from build123d import *

# Parameters (mm, degrees)
F0_R     = 54.998868
F1_DEPTH = 30
F2_R     = 49.998868
F2_R_2   = 48.998866
F3_DEPTH = 3
F4_R     = 49.998868
F4_R_2   = 48.998866
F5_DEPTH = 3


with BuildPart() as f1:
    # F0 (on Top) → F1 (new body)
    with BuildSketch(Plane.XY):
        Circle(F0_R)
    extrude(amount=F1_DEPTH)

    # F2 (on face) → F3 (join)
    with BuildSketch(Plane(origin=(0, 0, 0), x_dir=(1, 0, 0), z_dir=(0, 0, -1))):
        Circle(F2_R)
        Circle(F2_R_2, mode=Mode.SUBTRACT)
    extrude(amount=F3_DEPTH)

    # F4 (on face) → F5 (join)
    with BuildSketch(Plane.XY.offset(30)):
        Circle(F4_R)
        Circle(F4_R_2, mode=Mode.SUBTRACT)
    extrude(amount=F5_DEPTH)


solid = f1.part
The model under review builds one solid part; all positions refer to its coordinate system, in mm. A direction names the side the tool comes from. Give positions to 0.01 mm unless a question says otherwise; leave off trailing zeros. Loops run counter-clockwise (first coordinate to the right, second up) from the corner with the lowest first, then second, coordinate; pieces in that order, holes last. Notation, with made-up numbers: (-8.5, 43.25) -> (33.5, 43.25) arc R24 ccw to (33.5, 67.25) -> close; hole circle Ø2 at (77, 33). An arc over 180 degrees is marked (long way). Put each result on its own line as item: value. Start each with the question number.
1. Clearance check with flat-ended pins moving along their axes: P1, Ø1, axis at x = 9, z = 7, coming from the -Y side; P2, Ø12, axis at y = -25, z = 6.5, coming from the +X side; P3, Ø1, axis at y = -39, z = 3.5, coming from the +X side. State where each tip first meets the part, or that it passes through.
2. We need section A-A on y = 0. State the section outline as (x, z) points, then the cut area to 3 significant figures.
3. Wall thickness on probe 1 along Y at (x, z) = (0, -1); probe 2 along Z at (x, y) = (14, 38.5): over which ranges is each line inside the solid? List them lowest first.
4. We need section C-C on z = 26.5. State the section outline as (x, y) points, then the cut area to 3 significant figures.
5. For faces 1 (the face through (-1, 1, 30)), 2 (the face through (33, 37, -3)), 3 (the face through (12, -49, 0)), list the 3-axis set-ups (+Z, -Z, +X, -X, +Y, -Y) from which the entire face can be reached by the end or side of a thin tool; tool diameter is ignored.
6. Mouldability with a two-part tool opening along X and no side actions: class faces 4 (the face through (12, -49, 30)), 5 (the face through (-6.509, -49.573, -1.479)), 6 (the face through (-10.622, 47.834, -1.479)) as released by +X, released by -X, zero draft, split by the parting line, or undercut.
Determined:
1. P1: y = -54.34
1. P2: x = 51.61
1. P3: x = 39.28
2. outline: (-55, 0) -> (-50, 0) -> (-50, -3) -> (-49, -3) -> (-49, 0) -> (49, 0) -> (49, -3) -> (50, -3) -> (50, 0) -> (55, 0) -> (55, 30) -> (50, 30) -> (50, 33) -> (49, 33) -> (49, 30) -> (-49, 30) -> (-49, 33) -> (-50, 33) -> (-50, 30) -> (-55, 30) -> close
2. area: 3,310 mm^2
3. probe 1: -50 to -49, 49 to 50
3. probe 2: 0 to 30
4. outline: circle Ø110 at (0, 0)
4. area: 9,500 mm^2
5. face 1: +Z
5. face 2: -Z, +X, -X, +Y, -Y
5. face 3: -Z
6. face 4: zero draft
6. face 5: split by the parting line
6. face 6: undercut
